For this review, take the finished solid that the model builds, in its own axes (mm). A direction names the side the tool comes from. Give positions to 0.01 mm unless a question says otherwise; leave off trailing zeros. Use one line per item in the form item = value. Start each with the question number.
Q1. Clearance check with flat-ended pins moving along their axes: pin 1 Ø0.6 at (y, z) = (1.5, -12) entering from -X (3 decimals); pin 2 Ø1.5 at (x, z) = (-15.5, -5) entering from -Y; pin 3 Ø0.6 at (x, z) = (0.5, -12) entering from -Y (3 decimals). State where each tip first meets the part, or that it passes through.
Q2. Consider section B-B on x = 0. Give the number of separate pieces and of enclosed holes in the cut face, and give its area (3 significant figures).
Q3. Mouldability with a two-part tool opening along Y and no side actions: class faces 5 (the flat face through (20.955, 0, -5)), 6 (the cylindrical face through (0.133, 21.461, 1.816)), 7 (the flat face through (-20.955, 0, -5)), 8 (the flat face through (20.955, 0, -12)) as released by +Y, released by -Y, zero draft, split by the parting line, or undercut.
Q4. For probe 1 along Y at (x, z) = (0, -11.35) (3 decimals); probe 2 along Y at (x, z) = (0, -12.1) (3 decimals); probe 3 along Y at (x, z) = (-7, -7) (3 decimals), list the stretches that pass through material, from the lowest coordinate up. Write a range as [from, to].
Q5. Tool access review of faces 1 (the cylindrical face through (14.676, -14.791, -11.448)), 2 (the flat face through (-10, -9, 0)), 3 (the cylindrical face through (17.696, 17.518, -12.074)), 4 (the cylindrical face through (-17.518, 17.696, -12.074)): name each direction out of +Z, -Z, +X, -X, +Y, -Y from which nothing blocks a thin tool from reaching the whole face with its end or side.
```python
from build123d import *

# Parameters (mm, degrees)
BOSS_EXTRUDE1_DEPTH     = 2.54
SKETCH3_R               = 14.605
BOSS_EXTRUDE2_DEPTH     = 1.27
CUT_EXTRUDE1_DEPTH      = 32.66097519
CUT_EXTRUDE1_DEPTH_BACK = 32.66097519
SKETCH4_R               = 12.7
BOSS_EXTRUDE3_START     = 11.43
BOSS_EXTRUDE3_DEPTH     = 11.43
BOSS_EXTRUDE5_START     = 1.27
BOSS_EXTRUDE5_DEPTH     = 2.54
FILLET2_R               = 1.27
CUT_EXTRUDE2_DEPTH      = 36.503258301
CUT_EXTRUDE2_DEPTH_BACK = 36.503258301
SKETCH7_R               = 1.27
CHAMFER1_SIZE           = 1.27
FILLET3_R               = 2.54


# Some blends are built 0.0001 mm under size
with BuildPart() as part:
    # Sketch2 → Boss-Extrude1 (new body)
    with BuildSketch(Plane.XY):
        with BuildLine():
            Line((-9.525, -22.225), (9.525, -22.225))
            ThreePointArc((9.525, -22.225), (18.505256121, -18.505256121), (22.225, -9.525))
            Line((22.225, -9.525), (22.225, 9.525))
            ThreePointArc((22.225, 9.525), (18.505256121, 18.505256121), (9.525, 22.225))
            Line((9.525, 22.225), (-9.525, 22.225))
            ThreePointArc((-9.525, 22.225), (-18.505256121, 18.505256121), (-22.225, 9.525))
            Line((-22.225, 9.525), (-22.225, -9.525))
            ThreePointArc((-22.225, -9.525), (-18.505256121, -18.505256121), (-9.525, -22.225))
        make_face()
    extrude(amount=BOSS_EXTRUDE1_DEPTH)

    # Sketch3 → Boss-Extrude2 (add)
    with BuildSketch(Plane.XY.offset(2.54)):
        Circle(SKETCH3_R)
    extrude(amount=BOSS_EXTRUDE2_DEPTH)

    # Sketch4 → Cut-Extrude1 (cut, two sides: drawn at the far end of the back side and taken through both)
    with BuildSketch(Plane.XY.offset(3.81).offset(-CUT_EXTRUDE1_DEPTH_BACK)):
        Circle(SKETCH4_R)
    extrude(amount=CUT_EXTRUDE1_DEPTH + CUT_EXTRUDE1_DEPTH_BACK, mode=Mode.SUBTRACT)

    # Sketch5 → Boss-Extrude3 (add)
    with BuildSketch(Plane(origin=(0, 0, 0), x_dir=(-1, 0, 0), z_dir=(0, 0, -1)).offset(BOSS_EXTRUDE3_START)):
        with BuildLine():
            Line((-22.225, 9.525), (-22.225, -9.525))
            ThreePointArc((-22.225, -9.525), (-18.505256121, -18.505256121), (-9.525, -22.225))
            Line((-9.525, -22.225), (9.525, -22.225))
            ThreePointArc((9.525, -22.225), (18.505256121, -18.505256121), (22.225, -9.525))
            Line((22.225, -9.525), (22.225, 9.525))
            ThreePointArc((22.225, 9.525), (18.505256121, 18.505256121), (9.525, 22.225))
            Line((9.525, 22.225), (-9.525, 22.225))
            ThreePointArc((-9.525, 22.225), (-18.505256121, 18.505256121), (-22.225, 9.525))
        make_face()
        with BuildLine():
            Line((-9.525, 20.955), (9.525, 20.955))
            ThreePointArc((9.525, 20.955), (17.607230509, 17.607230509), (20.955, 9.525))
            Line((20.955, 9.525), (20.955, -9.525))
            ThreePointArc((20.955, -9.525), (17.607230509, -17.607230509), (9.525, -20.955))
            Line((9.525, -20.955), (-9.525, -20.955))
            ThreePointArc((-9.525, -20.955), (-17.607230509, -17.607230509), (-20.955, -9.525))
            Line((-20.955, -9.525), (-20.955, 9.525))
            ThreePointArc((-20.955, 9.525), (-17.607230509, 17.607230509), (-9.525, 20.955))
        make_face(mode=Mode.SUBTRACT)
    extrude(amount=-BOSS_EXTRUDE3_DEPTH)

    # Sketch6 → Boss-Extrude5 (add)
    with BuildSketch(Plane(origin=(0, 0, -11.43), x_dir=(-1, 0, 0), z_dir=(0, 0, -1)).offset(BOSS_EXTRUDE5_START)):
        with BuildLine():
            Line((-9.525, 20.955), (9.525, 20.955))
            ThreePointArc((9.525, 20.955), (17.607230509, 17.607230509), (20.955, 9.525))
            Line((20.955, 9.525), (20.955, -9.525))
            ThreePointArc((20.955, -9.525), (17.607230509, -17.607230509), (9.525, -20.955))
            Line((9.525, -20.955), (-9.525, -20.955))
            ThreePointArc((-9.525, -20.955), (-17.607230509, -17.607230509), (-20.955, -9.525))
            Line((-20.955, -9.525), (-20.955, 9.525))
            ThreePointArc((-20.955, 9.525), (-17.607230509, 17.607230509), (-9.525, 20.955))
        make_face()
        with BuildLine():
            Line((-9.525, 16.891), (9.525, 16.891))
            ThreePointArc((9.525, 16.891), (14.73354855, 14.73354855), (16.891, 9.525))
            Line((16.891, 9.525), (16.891, -9.525))
            ThreePointArc((16.891, -9.525), (14.73354855, -14.73354855), (9.525, -16.891))
            Line((9.525, -16.891), (-9.525, -16.891))
            ThreePointArc((-9.525, -16.891), (-14.73354855, -14.73354855), (-16.891, -9.525))
            Line((-16.891, -9.525), (-16.891, 9.525))
            ThreePointArc((-16.891, 9.525), (-14.73354855, 14.73354855), (-9.525, 16.891))
        make_face(mode=Mode.SUBTRACT)
    extrude(amount=-BOSS_EXTRUDE5_DEPTH)

    # Fillet2
    fillet2_edges = [part.edges().sort_by_distance(p)[0] for p in [
        (-14.605, 0, 2.54),
        (-12.7, 0, 3.81),
    ]]
    fillet(fillet2_edges, radius=FILLET2_R - 0.0001)  # a hair under: the kernel refuses the full size

    # Sketch7 → Cut-Extrude2 (cut, two sides: drawn at the far end of the back side and taken through both)
    with BuildSketch(Plane(origin=(0, 0, -12.7), x_dir=(-1, 0, 0), z_dir=(0, 0, -1)).offset(-CUT_EXTRUDE2_DEPTH_BACK)):
        with Locations((0, 18.923)):
            Circle(SKETCH7_R)
        with Locations((0, -18.923)):
            Circle(SKETCH7_R)
    extrude(amount=CUT_EXTRUDE2_DEPTH + CUT_EXTRUDE2_DEPTH_BACK, mode=Mode.SUBTRACT)

    # Chamfer1
    chamfer1_edges = [part.edges().sort_by_distance(p)[0] for p in [
        (1.27, 18.923, 2.54),
        (1.27, -18.923, 2.54),
    ]]
    chamfer(chamfer1_edges, length=CHAMFER1_SIZE)

    # Fillet3
    # the kernel refuses this fillet: 2.54 mm, written as the material it takes off along each edge
    with BuildSketch(Plane(origin=(9.525, -9.525, 2.54), x_dir=(0, -1, 0), z_dir=(-1, 0, 0))) as fillet3_piece_1:
        with BuildLine():
            CenterArc((12.7 - FILLET3_R, -FILLET3_R), FILLET3_R, 0, 90)
            Line((12.7, -FILLET3_R), (12.7, 0))
            Line((12.7, 0), (12.7 - FILLET3_R, 0))
        make_face()
    revolve(axis=Axis((9.525, -9.525, 2.54), (0, 0, 1)), revolution_arc=90, mode=Mode.SUBTRACT)
    with BuildSketch(Plane(origin=(22.225, -9.525, 2.54), x_dir=(-1, 0, 0), z_dir=(0, 1, 0)), Plane(origin=(9.525, 22.225, 2.54), x_dir=(0, -1, 0), z_dir=(-1, 0, 0)), Plane(origin=(-22.225, 9.525, 2.54), x_dir=(1, 0, 0), z_dir=(0, -1, 0)), Plane(origin=(-9.525, -22.225, 2.54), x_dir=(0, 1, 0), z_dir=(1, 0, 0))) as fillet3_piece_2:
        with BuildLine():
            CenterArc((FILLET3_R, -FILLET3_R), FILLET3_R, 90, 90)
            Line((0, -FILLET3_R), (0, 0))
            Line((0, 0), (FILLET3_R, 0))
        make_face()
    extrude(amount=19.05, mode=Mode.SUBTRACT)
    with BuildSketch(Plane(origin=(9.525, 9.525, 2.54), x_dir=(1, 0, 0), z_dir=(0, -1, 0))) as fillet3_piece_3:
        with BuildLine():
            CenterArc((12.7 - FILLET3_R, -FILLET3_R), FILLET3_R, 0, 90)
            Line((12.7, -FILLET3_R), (12.7, 0))
            Line((12.7, 0), (12.7 - FILLET3_R, 0))
        make_face()
    revolve(axis=Axis((9.525, 9.525, 2.54), (0, 0, 1)), revolution_arc=90, mode=Mode.SUBTRACT)
    with BuildSketch(Plane(origin=(-9.525, 9.525, 2.54), x_dir=(0, 1, 0), z_dir=(1, 0, 0))) as fillet3_piece_4:
        with BuildLine():
            CenterArc((12.7 - FILLET3_R, -FILLET3_R), FILLET3_R, 0, 90)
            Line((12.7, -FILLET3_R), (12.7, 0))
            Line((12.7, 0), (12.7 - FILLET3_R, 0))
        make_face()
    revolve(axis=Axis((-9.525, 9.525, 2.54), (0, 0, 1)), revolution_arc=90, mode=Mode.SUBTRACT)
    with BuildSketch(Plane(origin=(-9.525, -9.525, 2.54), x_dir=(-1, 0, 0), z_dir=(0, 1, 0))) as fillet3_piece_5:
        with BuildLine():
            CenterArc((12.7 - FILLET3_R, -FILLET3_R), FILLET3_R, 0, 90)
            Line((12.7, -FILLET3_R), (12.7, 0))
            Line((12.7, 0), (12.7 - FILLET3_R, 0))
        make_face()
    revolve(axis=Axis((-9.525, -9.525, 2.54), (0, 0, 1)), revolution_arc=90, mode=Mode.SUBTRACT)


solid = part.part
```
Working result:
q1.pin_1 = -20.955
q1.pin_2 = -21.1
q1.pin_3 = -20.955
q2.separate_pieces = 6
q2.enclosed_holes = 0
q2.area = 71.6 mm²
q3.face_5 = undercut
q3.face_6 = released by +Y
q3.face_7 = undercut
q3.face_8 = zero draft
q4.probe_1 = [-22.225, -20.193], [-17.653, -16.891], [16.891, 17.653], [20.193, 22.225]
q4.probe_2 = [-20.955, -20.193], [-17.653, -16.891], [16.891, 17.653], [20.193, 20.955]
q4.probe_3 = [-22.225, -20.955], [20.955, 22.225]
q5.face_1 = -Z
q5.face_2 = none
q5.face_3 = -Z, +X, +Y
q5.face_4 = -Z, -X, +Y
